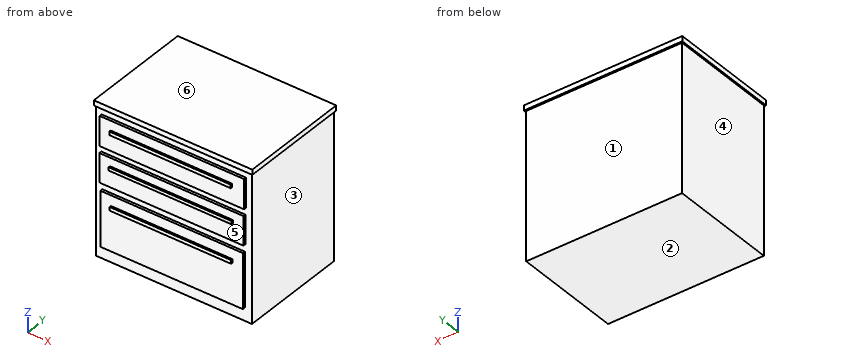
from build123d import *

# Parameters (mm, degrees)
F0_W      = 548.64
F0_H      = 381
F1_DEPTH  = 518.16
F2_W      = 558.0791532993
F2_H      = 390.8702135086
F2_W_2    = 548.64
F2_H_2    = 381
F3_DEPTH  = 17.9832
F4_W      = 508.8175535202
F4_H      = 104.0762960911
F5_W      = 507.6611340046
F5_H      = 101.7635166645
F6_W      = 501.8791407347
F6_H      = 193.1193843484
F7_DEPTH  = 9.144
F10_W     = 427.862867713
F10_H     = 12.6414000988
F9_W      = 433.3813935518
F9_H      = 11.4478170872
F8_W      = 427.6882261038
F8_H      = 12.3768150806
F11_DEPTH = 6.096


with BuildPart() as f1:
    # F0 (on Top) → F1 (new body)
    with BuildSketch(Plane.XY):
        Rectangle(F0_W, F0_H)
    extrude(amount=F1_DEPTH)

    # F2 (on face) → F3 (join)
    with BuildSketch(Plane.XY.offset(518.16)):
        with Locations((-0.2440661192, 0.519618392)):
            Rectangle(F2_W, F2_H)
        Rectangle(F2_W_2, F2_H_2, mode=Mode.SUBTRACT)
        Rectangle(F2_W_2, F2_H_2)
    extrude(amount=F3_DEPTH)

    # F4 (on face) + F5 (on face) + F6 (on face) → F7 (join)
    with BuildSketch(Plane.XZ.offset(190.5)):
        with Locations((-0.822275877, 443.328037858)):
            Rectangle(F4_W, F4_H)
    with BuildSketch(Plane.XZ.offset(190.5)):
        with Locations((-2.5568753481, 316.123649478)):
            Rectangle(F5_W, F5_H)
    with BuildSketch(Plane.XZ.offset(190.5)):
        with Locations((-1.9786730409, 142.0849226415)):
            Rectangle(F6_W, F6_H)
    extrude(amount=F7_DEPTH)

    # F10 (on face) + F9 (on face) + F8 (on face) → F11 (join)
    with BuildSketch(Plane.XZ.offset(199.644)):
        with Locations((-1.7024800181, 195.7238912582)):
            Rectangle(F10_W, F10_H)
    with BuildSketch(Plane.XZ.offset(199.644)):
        with Locations((-2.1058097482, 331.7696303129)):
            Rectangle(F9_W, F9_H)
    with BuildSketch(Plane.XZ.offset(199.644)):
        with Locations((-2.7256086469, 455.3973823786)):
            Rectangle(F8_W, F8_H)
    extrude(amount=F11_DEPTH)


solid = f1.part
Build history of the part. All positions in model axes, mm. Face numbers are marked on the shaded views. A direction names the side the tool comes from. Coordinates: 2 decimals unless noted, no trailing zeros. Write each loop counter-clockwise with the first axis right and the second up, starting at its lowest first coordinate (ties: lowest second). Pieces come first, ordered by that corner, then holes. Notation, with made-up numbers: (-35.75, 44) -> (-22.75, 44) arc R10 cw to (-22.75, 61) -> close; hole circle Ø1 at (15, 39). An arc over 180 degrees is marked (long way). Use CSV: the item, a comma, the result in double quotes. Start each with the question number.
Q1. Cut at B-B, the plane y = -133.5. List the corners of the cut face in (x, z), then the cut area to 3 significant figures.
Q2. Pull direction Z, two halves, no side cores. Call the marked faces 4, 5 and 6: released by +Z, released by -Z, zero draft, split by the parting line, or undercut.
Q3. Flat gauge pins, fed straight in: pin 1 Ø1.8 at (x, y) = (53, -203.5) entering from +Z; pin 2 Ø10 at (y, z) = (-194, 325.5) entering from -X; pin 3 Ø8 at (y, z) = (16, 184) entering from +X. Where does each tip first touch, or does it go through?
Q4. Cut at C-C, the plane z = 404.5. List the corners of the cut face in (x, y), then the cut area to 3 significant figures.
Q5. Drill centre lines: probe 1 along X at (y, z) = (152, 143.5); probe 2 along Y at (x, z) = (-199, 278.5); probe 3 along Y at (x, z) = (93, 511). Where is each one in solid material? Low to high.
Q6. Cut at D-D, the plane z = 251. List the corners of the cut face in (x, y), then the cut area to 3 significant figures.
Q7. 3-axis set-ups, long thin cutter, end or side, ignore diameter. For the marked faces 1, 2 and 3: which of +Z, -Z, +X, -X, +Y, -Y reach the whole face in a straight line?
Checked values:
1,outline,"(-279.28, 518.16) -> (-274.32, 518.16) -> (-274.32, 0) -> (274.32, 0) -> (274.32, 518.16) -> (278.8, 518.16) -> (278.8, 536.14) -> (-279.28, 536.14) -> close"
1,area,"294,000 mm²"
2,face 4,"zero draft"
2,face 5,"undercut"
2,face 6,"released by +Z"
3,pin 1,"stops at z = 461.59"
3,pin 2,"stops at x = -274.32"
3,pin 3,"stops at x = 274.32"
4,outline,"(-274.32, -190.5) -> (-255.23, -190.5) -> (-255.23, -199.64) -> (253.59, -199.64) -> (253.59, -190.5) -> (274.32, -190.5) -> (274.32, 190.5) -> (-274.32, 190.5) -> close"
4,area,"214,000 mm²"
5,probe 1,"x = -274.32 to 274.32"
5,probe 2,"y = -199.64 to 190.5"
5,probe 3,"y = -190.5 to 190.5"
6,outline,"(-274.32, -190.5) -> (274.32, -190.5) -> (274.32, 190.5) -> (-274.32, 190.5) -> close"
6,area,"209,000 mm²"
7,face 1,"-Z, +X, -X, +Y"
7,face 2,"-Z, +X, -X, +Y, -Y"
7,face 3,"-Z, +X, +Y, -Y"
